Verification items for the finished model (mm, model axes). A direction names the side the tool comes from. Coordinates: 2 decimals unless noted, no trailing zeros. Order: outer loops, then holes, each group sorted by start corner. A loop starts at its lowest first (then second) coordinate and runs counter-clockwise, first axis right, second up.
Q1. Cross-section at A-A, the plane z = 23.25. Record the boundary of the cut face in (x, y).
Q2. Thickness scan on line 1 (Z direction, x = -5.75, y = -13.25); line 2 (X direction, y = -2.25, z = 17.5); line 3 (X direction, y = -16.5, z = 25.75). Record the ranges inside material, lowest first.
Q3. Cross-section at D-D, the plane x = -3. Record the boundary of the cut face in (y, z), and give its area (3 significant figures).
Q4. Cross-section at C-C, the plane y = -17. Record the boundary of the cut face in (x, z).
Q5. Set-up check for faces 1 (the flat face through (-3, -16, 22.271)), 2 (the cylindrical face through (5.458, 4.175, 19.106)), 3 (the flat face through (-3, -16, 32.271)): record each of +Z, -Z, +X, -X, +Y, -Y from which the full face is reachable in a straight line by a thin tool's end or side.
Q6. Cross-section at B-B, the plane x = 2. Record the boundary of the cut face in (y, z).
Q7. Depth check by flat-ended pin: P1, Ø3.5, axis at x = -3.5, z = 28, coming from the +Y side; P2, Ø8, axis at y = 4, z = 35.5, coming from the +X side; P3, Ø2, axis at y = 0.5, z = 36.5, coming from the -X side. Enter the tip coordinate at first touch or a pass-through.
from build123d import *

# Parameters (mm, degrees)
SKETCH1_W           = 27
SKETCH1_H           = 27
BOSS_EXTRUDE1_DEPTH = 2.5
SKETCH2_R           = 1.25
BOSS_EXTRUDE2_DEPTH = 6
SKETCH3_W           = 10
SKETCH3_H           = 6
BOSS_EXTRUDE3_DEPTH = 7
CUT_EXTRUDE1_DEPTH  = 10.5


with BuildPart() as part:
    # Sketch1 → Boss-Extrude1 (new body)
    with BuildSketch(Plane(origin=(0, 0, 0), x_dir=(0, 0, -1), z_dir=(1, 0, 0))):
        with Locations((-28.770960436, -5.47612775)):
            Rectangle(SKETCH1_W, SKETCH1_H)
    extrude(amount=BOSS_EXTRUDE1_DEPTH)

    # Sketch2 → Boss-Extrude2 (add)
    with BuildSketch(Plane(origin=(2.5, 0, 0), x_dir=(0, 0, -1), z_dir=(1, 0, 0))):
        with Locations((-20.260960436, 4.65387225)):
            Circle(SKETCH2_R)
    extrude(amount=BOSS_EXTRUDE2_DEPTH)

    # Sketch3 → Boss-Extrude3 (add)
    with BuildSketch(Plane.ZY):
        with Locations((27.270960436, -15.97612775)):
            Rectangle(SKETCH3_W, SKETCH3_H)
    extrude(amount=BOSS_EXTRUDE3_DEPTH)

    # Sketch4 → Cut-Extrude1 (cut, through all)
    with BuildSketch(Plane(origin=(2.5, 0, 0), x_dir=(0, 0, -1), z_dir=(1, 0, 0))):
        Polygon((-42.270960436, -5.47612775), (-28.770960436, 8.02387225), (-42.270960436, 8.02387225), align=None)
    extrude(amount=-CUT_EXTRUDE1_DEPTH, mode=Mode.SUBTRACT)


solid = part.part
Check values:
1. outline: (-7, -18.98) - (2.5, -18.98) - (2.5, 8.02) - (0, 8.02) - (0, -12.98) - (-7, -12.98) - close
2. line 1: z = 22.27 to 32.27
2. line 2: x = 0 to 2.5
2. line 3: x = -7 to 2.5
3. outline: (-18.98, 22.27) - (-12.98, 22.27) - (-12.98, 32.27) - (-18.98, 32.27) - close
3. area: 60.0 mm2
4. outline: (-7, 22.27) - (0, 22.27) - (0, 15.27) - (2.5, 15.27) - (2.5, 42.27) - (0, 42.27) - (0, 32.27) - (-7, 32.27) - close
5. face 1: -Z, -X, +Y, -Y
5. face 2: +X
5. face 3: +Z, -X, +Y, -Y
6. outline: (-18.98, 15.27) - (8.02, 15.27) - (8.02, 28.77) - (-5.48, 42.27) - (-18.98, 42.27) - close
7. P1: stops at y = -12.98
7. P2: stops at x = 2.5
7. P3: stops at x = 0
